```python
from build123d import *

# Parameters (mm, degrees)
SKETCH1_R               = 120
BOSS_EXTRUDE1_DEPTH     = 10
CUT_EXTRUDE1_DEPTH      = 171
CUT_EXTRUDE1_DEPTH_BACK = 171
SKETCH2_R               = 10
CUT_EXTRUDE2_DEPTH      = 171
CUT_EXTRUDE2_DEPTH_BACK = 171
SKETCH3_R               = 10
SKETCH8_W               = 35
SKETCH8_H               = 50
BOSS_EXTRUDE3_DEPTH     = 5
SKETCH9_W               = 50
SKETCH9_H               = 45
BOSS_EXTRUDE4_DEPTH     = 5
SKETCH10_W              = 105
SKETCH10_H              = 50
BOSS_EXTRUDE5_DEPTH     = 5
SKETCH11_R              = 5
CUT_EXTRUDE3_DEPTH      = 176.570498661
SKETCH12_R              = 7.5
BOSS_EXTRUDE6_DEPTH     = 2.5


with BuildPart() as part:
    # Sketch1 → Boss-Extrude1 (new body)
    with BuildSketch(Plane(origin=(0, 0, 0), x_dir=(1, 0, 0), z_dir=(0, 1, 0))):
        with Locations(Location((0, 0, 0), (0, 0, 270))):
            Circle(SKETCH1_R)
    extrude(amount=BOSS_EXTRUDE1_DEPTH)

    # Sketch2 → Cut-Extrude1 (cut, two sides: drawn at the far end of the back side and taken through both)
    with BuildSketch(Plane(origin=(0, 10, 0), x_dir=(1, 0, 0), z_dir=(0, 1, 0)).offset(-CUT_EXTRUDE1_DEPTH_BACK)):
        with Locations(Location((0, 0, 0), (0, 0, 270))):
            Circle(SKETCH2_R)
    extrude(amount=CUT_EXTRUDE1_DEPTH + CUT_EXTRUDE1_DEPTH_BACK, mode=Mode.SUBTRACT)

    # Sketch3 → Cut-Extrude2 (cut, two sides: drawn at the far end of the back side and taken through both)
    with BuildSketch(Plane(origin=(0, 10, 0), x_dir=(1, 0, 0), z_dir=(0, 1, 0)).offset(-CUT_EXTRUDE2_DEPTH_BACK)):
        with Locations(Location((0, 100, 0), (0, 0, 270))):
            Circle(SKETCH3_R)
        with Locations(Location((-70, -75, 0), (0, 0, 270))):
            Circle(SKETCH3_R)
        with Locations(Location((70, -75, 0), (0, 0, 90))):
            Circle(SKETCH3_R)
    extrude(amount=CUT_EXTRUDE2_DEPTH + CUT_EXTRUDE2_DEPTH_BACK, mode=Mode.SUBTRACT)

    # Sketch8 → Boss-Extrude3 (add)
    with BuildSketch(Plane(origin=(0, 10, 0), x_dir=(1, 0, 0), z_dir=(0, 1, 0))):
        with Locations((-70, -0.262373312)):
            Rectangle(SKETCH8_W, SKETCH8_H)
    boss_extrude3 = extrude(amount=BOSS_EXTRUDE3_DEPTH)

    # Mirror2: Boss-Extrude3 across plane
    add(boss_extrude3.mirror(Plane(origin=(0, 0, 0), x_dir=(0, 0, 1), z_dir=(1, 0, 0))))

    # Sketch9 → Boss-Extrude4 (add)
    with BuildSketch(Plane(origin=(-52.5, 0, 0), x_dir=(0, 0, -1), z_dir=(1, 0, 0))):
        with Locations((-0.262373312, 32.5)):
            Rectangle(SKETCH9_W, SKETCH9_H)
    boss_extrude4 = extrude(amount=BOSS_EXTRUDE4_DEPTH)

    # Mirror3: Boss-Extrude4 across plane
    add(boss_extrude4.mirror(Plane(origin=(0, 0, 0), x_dir=(0, 0, 1), z_dir=(1, 0, 0))))

    # Sketch10 → Boss-Extrude5 (add)
    with BuildSketch(Plane(origin=(0, 55, 0), x_dir=(1, 0, 0), z_dir=(0, 1, 0))):
        with Locations((0, -0.262373312)):
            Rectangle(SKETCH10_W, SKETCH10_H)
    extrude(amount=BOSS_EXTRUDE5_DEPTH)

    # Sketch11 → Cut-Extrude3 (cut, symmetric)
    with BuildSketch(Plane(origin=(0, 15, 0), x_dir=(1, 0, 0), z_dir=(0, 1, 0))):
        with Locations(Location((-72.5, 17.904853765, 0), (0, 0, 270))):
            Circle(SKETCH11_R)
        with Locations(Location((-72.5, -16.970687481, 0), (0, 0, 270))):
            Circle(SKETCH11_R)
    cut_extrude3 = extrude(amount=CUT_EXTRUDE3_DEPTH, both=True, mode=Mode.SUBTRACT)

    # Mirror4: Cut-Extrude3 across plane
    add(cut_extrude3.mirror(Plane(origin=(0, 0, 0), x_dir=(0, 0, 1), z_dir=(1, 0, 0))), mode=Mode.SUBTRACT)

    # Sketch12 → Boss-Extrude6 (add)
    with BuildSketch(Plane(origin=(0, 15, 0), x_dir=(1, 0, 0), z_dir=(0, 1, 0))):
        with Locations(Location((-72.5, 17.904853765, 0), (0, 0, 114.351031906))):
            Circle(SKETCH12_R)
        with Locations(Location((-72.5, -17.904853765, 0), (0, 0, 90))):
            Circle(SKETCH12_R)
    boss_extrude6 = extrude(amount=BOSS_EXTRUDE6_DEPTH)

    # Mirror5: Boss-Extrude6 across plane
    add(boss_extrude6.mirror(Plane(origin=(0, 0, 0), x_dir=(0, 0, 1), z_dir=(1, 0, 0))))


solid = part.part
```
Geometry: final body of the model. Coordinates: model frame, mm. A direction names the side the tool comes from. Coordinates: 2 decimals unless noted, no trailing zeros. Order: outer loops, then holes, each group sorted by start corner. A loop starts at its lowest first (then second) coordinate and runs counter-clockwise, first axis right, second up. Notation, with made-up numbers: (44, 70.5) - (68, 70.5) arc R32 ccw to (68, 99.5) - close; hole circle Ø10 at (87.5, 6). An arc over 180 degrees is marked (long way). Write each question's results on one line, items separated by ' | '.
(1) Section query A-A, the plane y = 48.5. Return the cut outline in (x, z).
Values found:
outline: (-52.5, -24.74) - (-47.5, -24.74) - (-47.5, 25.26) - (-52.5, 25.26) - close; (47.5, -24.74) - (52.5, -24.74) - (52.5, 25.26) - (47.5, 25.26) - close
(2) Set-up query: faces 4 (the face through (73, 17.5, -18)), 5 (the face through (70.998, 7.605, -13.136)), 6 (the face through (-73, 17.5, 18)). Return all of +Z, -Z, +X, -X, +Y, -Y with unobstructed straight access to the full face (end or side cutting, diameter ignored); none if empty.
Values found:
face 4: +Z, -Z, +X, +Y | face 5: -Y | face 6: +Z, -Z, -X, +Y
(3) Section query D-D, the plane y = 5. Count the separate pieces of the cut face and the enclosed holes in it, plus the area to 3 significant figures.
Values found:
separate pieces: 1 | enclosed holes: 8 | area: 43,700 mm²
(4) Mould query, pull axis X, two halves, no side actions, for faces 1 (the face through (5.276, 4.93, -119.884)), 2 (the face through (2, 0, 25)), 3 (the face through (0, 5, -110)). Classes: +X half, -X half, draft (parallel to the pull), parting line (faces both ways), or undercut.
Values found:
face 1: parting line | face 2: draft | face 3: undercut
(5) Section query C-C, the plane z = -100. Return the cut outline in (x, y).
Values found:
outline: (-66.33, 0) - (-10, 0) - (-10, 10) - (-66.33, 10) - close; (10, 0) - (66.33, 0) - (66.33, 10) - (10, 10) - close
(6) First-contact query: pin 1 Ø10 at (x, y) = (-50, 14) entering from -Z; pin 2 Ø22.5 at (y, z) = (36, -6.5) entering from +X; pin 3 Ø12 at (x, z) = (73, -14.5) entering from +Y. Flat tips, straight axial feed; report the tip coordinate or a pass-through.
Values found:
pin 1: stops at z = -110.41 | pin 2: stops at x = 52.5 | pin 3: stops at y = 17.5
(7) Line query: line 1 (X direction, y = 3, z = 0); line 2 (Y direction, x = -13.5, z = 7.5); line 3 (X direction, y = 24, z = -11.5). Output: solid intervals per line, ascending. Write a range as [from, to].
Values found:
line 1: x = [-120, -10], [10, 120] | line 2: y = [0, 10], [55, 60] | line 3: x = [-52.5, -47.5], [47.5, 52.5]
(8) Section query B-B, the plane x = 0. Return the cut outline in (y, z), plus the area to 3 significant figures.
Values found:
outline: (0, -120) - (10, -120) - (10, -110) - (0, -110) - close; (0, -90) - (10, -90) - (10, -10) - (0, -10) - close; (0, 10) - (10, 10) - (10, 120) - (0, 120) - close; (55, -24.74) - (60, -24.74) - (60, 25.26) - (55, 25.26) - close | area: 2,250 mm²
